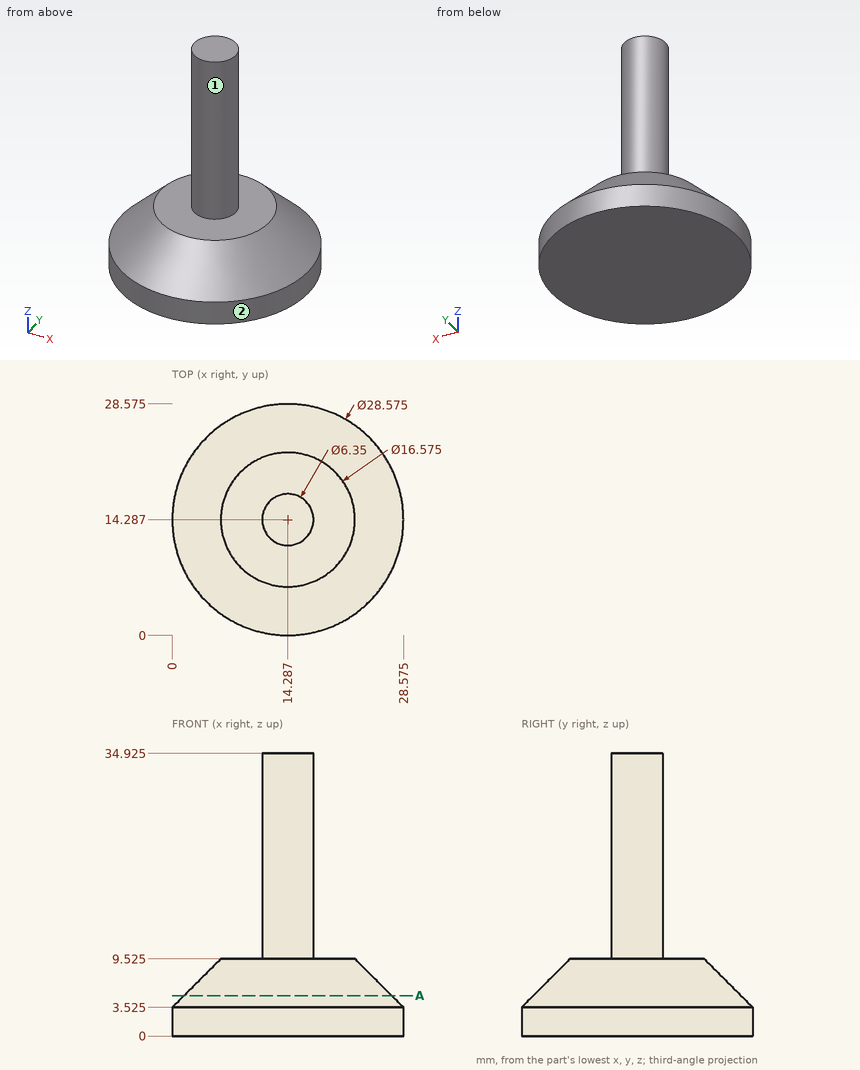
Part print with two shaded views. Sizes in mm from the minimum x, y, z corner. A direction names the side the tool comes from. Coordinates: 2 decimals unless noted, no trailing zeros. Order: outer loops, then holes, each group sorted by start corner. A loop starts at its lowest first (then second) coordinate and runs counter-clockwise, first axis right, second up. Notation, with made-up numbers: (66, -35.75) - (117, -35.75) arc R23 ccw to (117, -27.75) - close; hole circle Ø3 at (71.5, 30). An arc over 180 degrees is marked (long way). Answer in a Markdown table with one row per item.
1. Slice it at A-A, the plane z = 5. List the corners of the cut face in (x, y) (1 decimal), then the cut area to 3 significant figures.
Answer:
| item | result |
|---|---|
| outline | circle Ø25.6 at (14.3, 14.3) |
| area | 516 mm² |
2. Flat gauge pins, fed straight in: P1, Ø5, axis at y = 10, z = 31, coming from the -X side (1 decimal); P2, Ø3, axis at x = 18.5, z = 9, coming from the +Y side (1 decimal); P3, Ø1, axis at x = 15, z = 27.5, coming from the +Y side (1 decimal). Where does each tip first touch, or does it go through?
Answer:
| item | result |
|---|---|
| P1 | x = 11.7 |
| P2 | y = 23.8 |
| P3 | y = 17.5 |
3. Drill centre lines: L1, parallel to Z at x = 19.25, y = 19 (1 decimal); L2, parallel to Z at x = 9, y = 25 (1 decimal); L3, parallel to X at y = 12.75, z = 3. Where is each one in solid material? Low to high. Write a range as from..to.
Answer:
| item | result |
|---|---|
| L1 | 0..9.5 |
| L2 | 0..5.9 |
| L3 | 0.08..28.49 |
4. 3-axis set-ups, long thin cutter, end or side, ignore diameter. For the marked faces 1 and 2: which of +Z, -Z, +X, -X, +Y, -Y reach the whole face in a straight line?
Answer:
| item | result |
|---|---|
| face 1 | +Z |
| face 2 | +Z, -Z |
